For this review, take the finished solid that the model builds, in its own axes (mm). Give positions to 0.01 mm unless a question says otherwise; leave off trailing zeros. Order: outer loops, then holes, each group sorted by start corner. A loop starts at its lowest first (then second) coordinate and runs counter-clockwise, first axis right, second up. Notation, with made-up numbers: (14.5, -6) -> (36.5, -6) arc R15 cw to (36.5, 22) -> close; hole circle Ø8 at (75, 15). An arc over 180 degrees is marked (long way). Use CSV: the item, a comma, the result in double quotes. Start each with the question number.
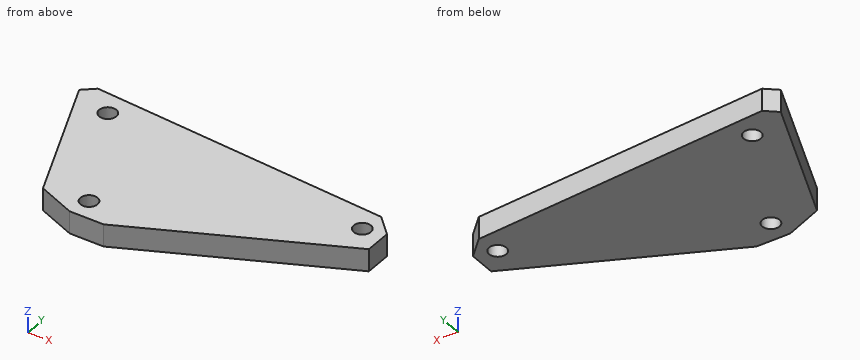
```python
from build123d import *
from OCP.BRepFilletAPI import BRepFilletAPI_MakeChamfer

# Parameters (mm, degrees)
BOSS_EXTRU_1_DEPTH           = 4
ENL_V_MAT_EXTRU_1_DEPTH      = 4
ENL_V_MAT_EXTRU_1_DEPTH_BACK = 7
ESQUISSE2_R                  = 1.55
CHANFREIN1_SIZE              = 3
CHANFREIN1_SIZE2             = 3.25880074
CHANFREIN1_SIZE2_2           = 5.532342211
CHANFREIN1_SIZE2_3           = 2.232526106


with BuildPart() as part:
    # Esquisse1 → Boss.-Extru.1 (new body)
    with BuildSketch(Plane.XY):
        Polygon((-19.694718841, 14.12522617), (-7.625402576, -15.080300035), (4.007307014, -15.080300035), (40.305281159, 1.726159227), (40.305281159, 9.522549697), align=None)
    extrude(amount=BOSS_EXTRU_1_DEPTH)

    # Esquisse2 → Enlèv. mat.-Extru.1 (cut, two sides: drawn at the far end of the back side and taken through both)
    with BuildSketch(Plane.XY.offset(4).offset(-ENL_V_MAT_EXTRU_1_DEPTH_BACK)):
        with Locations(Location((-11.887750079, 9.402917456, 0), (0, 0, 180))):
            Circle(ESQUISSE2_R)
        with Locations(Location((-1.222675499, -11.228701649, 0), (0, 0, 180))):
            Circle(ESQUISSE2_R)
        with Locations(Location((36.47491806, 5.624354462, 0), (0, 0, 180))):
            Circle(ESQUISSE2_R)
    extrude(amount=ENL_V_MAT_EXTRU_1_DEPTH + ENL_V_MAT_EXTRU_1_DEPTH_BACK, mode=Mode.SUBTRACT)

    # Chanfrein1: one chamfer whose edges measure the first distance from different faces: ONE call of the kernel's chamfer builder (chamfer() names one face for all edges)
    chanfrein1_edges_1 = [part.edges().sort_by_distance(p)[0] for p in [
        (40.305281159, 9.522549697, 2),
    ]]
    chanfrein1_side_1 = [part.faces().sort_by_distance(p)[0] for p in [
        (40.305281159, 5.624354462, 2),
    ]]
    chanfrein1_edges_2 = [part.edges().sort_by_distance(p)[0] for p in [
        (-7.625402576, -15.080300035, 2),
    ]]
    chanfrein1_side_2 = [part.faces().sort_by_distance(p)[0] for p in [
        (-13.660060709, -0.477536933, 2),
    ]]
    chanfrein1_edges_3 = [part.edges().sort_by_distance(p)[0] for p in [
        (-19.694718841, 14.12522617, 2),
    ]]
    chanfrein1_side_3 = [part.faces().sort_by_distance(p)[0] for p in [
        (10.305281159, 11.823887933, 2),
    ]]
    chanfrein1 = BRepFilletAPI_MakeChamfer(part.part.solid().wrapped)
    for e in chanfrein1_edges_1:
        chanfrein1.Add(CHANFREIN1_SIZE, CHANFREIN1_SIZE2, e.wrapped, chanfrein1_side_1[0].wrapped)  # the first distance lies on this face
    for e in chanfrein1_edges_2:
        chanfrein1.Add(CHANFREIN1_SIZE, CHANFREIN1_SIZE2_2, e.wrapped, chanfrein1_side_2[0].wrapped)  # the first distance lies on this face
    for e in chanfrein1_edges_3:
        chanfrein1.Add(CHANFREIN1_SIZE, CHANFREIN1_SIZE2_3, e.wrapped, chanfrein1_side_3[0].wrapped)  # the first distance lies on this face
    add(Compound.cast(chanfrein1.Shape()), mode=Mode.REPLACE)


solid = part.part
```
1. To check wall thickness, follow L1, parallel to X at y = 8, z = 0.3; L2, parallel to X at y = 6.5, z = 0.2; L3, parallel to Y at x = 23, z = 1.9. State the ranges of each line that lie inside material, in increasing order. Write a range as [from, to].
2. Consider section D-D (y = -7). State the section outline as (x, z) points.
3. Consider section C-C (x = 15.5). State the section outline as (y, z) points.
4. Consider section A-A (y = 5). State the section outline as (x, z) points.
5. Clearance check with flat-ended pins moving along their axes: P1, Ø1.5, axis at x = -7.5, z = 2.5, coming from the -Y side; P2, Ø1.5, axis at x = -12, z = 3.5, coming from the +Y side. State where each tip first meets the part, or that it passes through.
6. Consider section B-B (z = 1.1). State the section outline as (x, y) points, plus the area to 3 significant figures.
Answer list:
1,L1,"[-17.16, -12.55], [-11.23, 38.83]"
1,L2,"[-16.54, 35.2], [37.75, 40.31]"
1,L3,"[-6.29, 10.85]"
2,outline,"(-10.96, 0) -> (21.46, 0) -> (21.46, 4) -> (-10.96, 4) -> close"
3,outline,"(-9.76, 0) -> (11.43, 0) -> (11.43, 4) -> (-9.76, 4) -> close"
4,outline,"(-15.92, 0) -> (35.06, 0) -> (35.06, 4) -> (-15.92, 4) -> close; (37.89, 0) -> (40.31, 0) -> (40.31, 4) -> (37.89, 4) -> close"
5,P1,"y = -13.15"
5,P2,"y = 13.59"
6,outline,"(-18.84, 12.06) -> (-8.77, -12.31) -> (-2.09, -15.08) -> (4.01, -15.08) -> (40.31, 1.73) -> (40.31, 6.52) -> (37.06, 9.77) -> (-16.7, 13.9) -> close; hole circle Ø3.1 at (-11.89, 9.4); hole circle Ø3.1 at (-1.22, -11.23); hole circle Ø3.1 at (36.47, 5.62)"
6,area,"1,090 mm2"
